Source: three-view drawing plus pictorial views. Frame: mm from the lowest corner of the part. A direction names the side the tool comes from. Coordinates: 2 decimals unless noted, no trailing zeros. Write each loop counter-clockwise with the first axis right and the second up, starting at its lowest first coordinate (ties: lowest second). Pieces come first, ordered by that corner, then holes. Notation, with made-up numbers: (58.5, 71.5) -> (63.5, 71.5) arc R30 cw to (63.5, 98.5) -> close; hole circle Ø6 at (50, 35.25). An arc over 180 degrees is marked (long way). One line per item, written item: value. Start each with the question number.
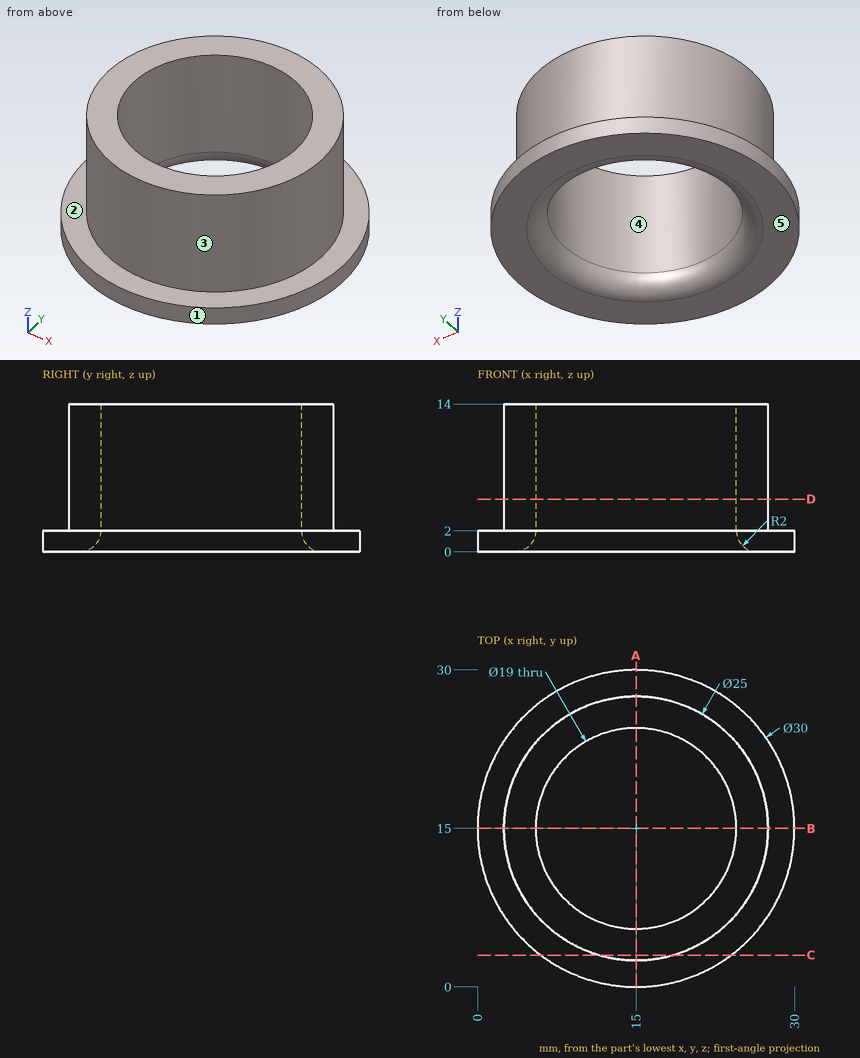
Q1. Cut plane D-D on z = 5. Output: boundary loops of the cut face in (x, y), and give its area (3 significant figures).
Q2. Access query for the marked faces 1 and 2. Directions: +Z, -Z, +X, -X, +Y, -Y. A direction counts if a zero-diameter tool reaches every point of the face in a straight line with its end or side. Return the directions, or none.
Q3. First-contact query: P1, Ø2, axis at y = 4, z = 9.5, coming from the -X side; P2, Ø6, axis at x = 22, z = 7.5, coming from the -Y side; P3, Ø3, axis at x = 10, z = 2, coming from the -Y side. Flat tips, straight axial feed; report the tip coordinate or a pass-through.
Q4. Cut plane C-C on y = 3. Output: boundary loops of the cut face in (x, z).
Q5. Cut plane A-A on x = 15. Output: boundary loops of the cut face in (y, z), and give its area (3 significant figures).
Q6. Line query: L1, parallel to Y at x = 15, z = 9; L2, parallel to Z at x = 4.75, y = 4.25; L3, parallel to X at y = 15.5, z = 9.25. Output: solid intervals per line, ascending. Write a range as from..to.
Q7. Draft query along X for the marked faces 3, 4 and 5. Return one class per face: pulls with the +X half, pulls with the -X half, needs draft (parallel to the pull), parting line crosses it, or undercut.
Solution:
1. outline: circle Ø25 at (15, 15); hole circle Ø19 at (15, 15)
1. area: 207 mm²
2. face 1: +Z, -Z
2. face 2: +Z
3. P1: x = 7.5
3. P2: y = 3.16
3. P3: y = 0.41
4. outline: (6, 0) -> (24, 0) -> (24, 2) -> (18.5, 2) -> (18.5, 14) -> (11.5, 14) -> (11.5, 2) -> (6, 2) -> close
5. outline: (0, 0) -> (3.5, 0) arc R2 ccw to (5.5, 2) -> (5.5, 14) -> (2.5, 14) -> (2.5, 2) -> (0, 2) -> close; (24.5, 2) arc R2 ccw to (26.5, 0) -> (30, 0) -> (30, 2) -> (27.5, 2) -> (27.5, 14) -> (24.5, 14) -> close
5. area: 92.3 mm²
6. L1: 2.5..5.5, 24.5..27.5
6. L2: 0..2
6. L3: 2.51..5.51, 24.49..27.49
7. face 3: parting line crosses it
7. face 4: undercut
7. face 5: needs draft
